Study the drawing (mm; zero at the part's minimum x, y, z) and answer. A direction names the side the tool comes from. Round coordinates to 2 decimals unless told otherwise and drop trailing zeros. Loops run counter-clockwise (first coordinate to the right, second up) from the corner with the lowest first, then second, coordinate; pieces in that order, holes last. Notation, with made-up numbers: (33, 36.25) -> (46, 36.25) arc R21 cw to (46, 70.25) -> close; hole circle Ø2 at (54.25, 39). An arc over 180 degrees is marked (long way). Write each question's results on one line, items separated by ' | '. Start each with the question number.
(1) The part is cut by section B-B (x = 99). Determine the outline of the cut face in (y, z), plus the area to 3 significant figures.
(2) For the marked faces 1, 2 and 3, determine the directions among +Z, -Z, +X, -X, +Y, -Y from which every point of the face is accessible in a straight line to the end or side of a thin tool.
(3) Straight lines are drawn through the part: probe 1 along X at (y, z) = (21, 4.75); probe 2 along X at (y, z) = (21, 6.5); probe 3 along Y at (x, z) = (99, 7.5). For each, find the intervals that lie inside material, in ascending order.
(4) Flat-ended cylindrical pins translate along their axes: pin 1 (1.5 mm diameter, centred on x = 70.5, z = 6.5, fed in from +Y); pin 2 (1 mm diameter, centred on y = 27, z = 8, fed in from -X); pin 3 (4 mm diameter, centred on y = 23.5, z = 4, fed in from +X); pin 4 (10 mm diameter, centred on x = 26, y = 14, fed in from -Z). Find the tip coordinate at first contact, or state that the pin passes through.
(5) The part is cut by section C-C (y = 23). Determine the outline of the cut face in (x, z).
(6) The part is cut by section A-A (z = 5). Determine the outline of the cut face in (x, y).
(7) The part is cut by section D-D (y = 31). Determine the outline of the cut face in (x, z), plus the area to 3 significant figures.
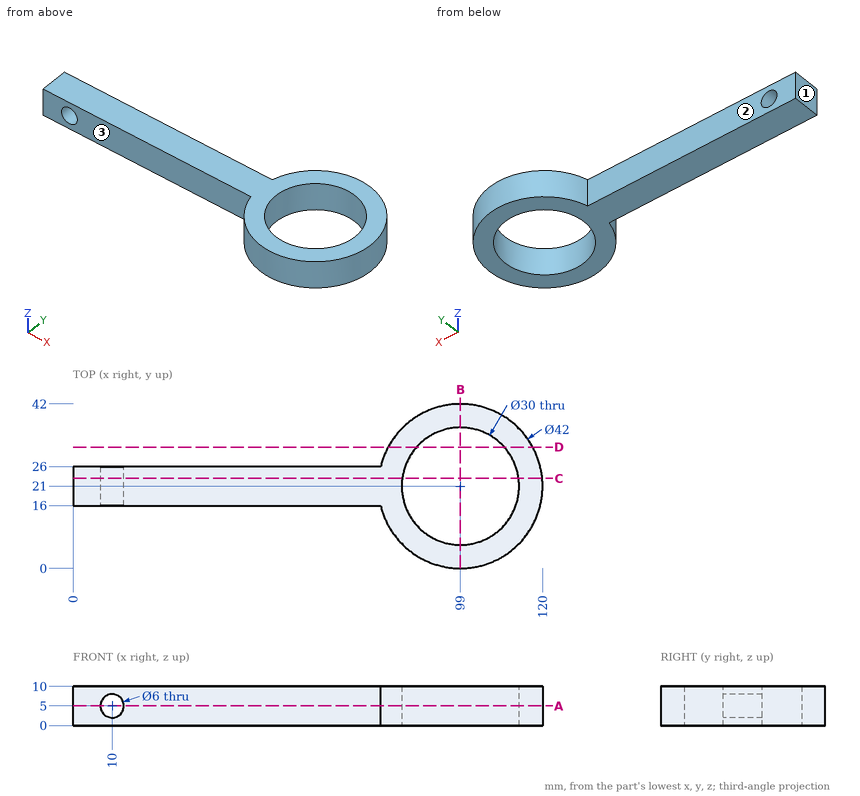
Checked values:
1) outline: (0, 0) -> (6, 0) -> (6, 10) -> (0, 10) -> close; (36, 0) -> (42, 0) -> (42, 10) -> (36, 10) -> close | area: 120 mm2
2) face 1: +Z, -Z, -X, +Y, -Y | face 2: +Z, -Z, -X, +Y | face 3: +Z, -Z, -X, -Y
3) probe 1: x = 0 to 7.01, 12.99 to 84, 114 to 120 | probe 2: x = 0 to 7.4, 12.6 to 84, 114 to 120 | probe 3: y = 0 to 6, 36 to 42
4) pin 1: stops at y = 26 | pin 2: stops at x = 78.73 | pin 3: stops at x = 119.99 | pin 4: stops at z = 0
5) outline: (0, 0) -> (84.13, 0) -> (84.13, 10) -> (0, 10) -> close; (113.87, 0) -> (119.9, 0) -> (119.9, 10) -> (113.87, 10) -> close; hole circle Ø6 at (10, 5)
6) outline: (0, 16) -> (7, 16) -> (7, 26) -> (0, 26) -> close; (13, 16) -> (78.6, 16) arc R21 ccw (long way) to (78.6, 26) -> (13, 26) -> close; hole circle Ø30 at (99, 21)
7) outline: (80.53, 0) -> (87.82, 0) -> (87.82, 10) -> (80.53, 10) -> close; (110.18, 0) -> (117.47, 0) -> (117.47, 10) -> (110.18, 10) -> close | area: 146 mm2
